Could you check a few things on this model? Use its own coordinates, in mm. A direction names the side the tool comes from. Coordinates: 2 decimals unless noted, no trailing zeros. Write each loop counter-clockwise with the first axis right and the second up, starting at its lowest first coordinate (ties: lowest second). Pieces come first, ordered by that corner, then holes. Notation, with made-up numbers: (82.25, -23) - (136.25, -23) arc R21 cw to (136.25, 15) - close; hole circle Ø8 at (50, 17). An arc over 180 degrees is marked (long way). Answer as a JSON object with one key per item and string values. Group by question number.
1) If we section it at B-B (y = 3): Write out the boundary of the cut face in (x, z).
2) Please list where these lines run through material, in increasing order: line 1 along Y through (x, z) = (-12.7, 138); line 2 along X through (y, z) = (-51, 87.5); line 3 along X through (y, z) = (-5, 118).
3) We'd pull the mould along Y, two halves only. Please class faces 1 (the flat face through (-24.3, -5.7, 38.1)), 2 (the flat face through (17.128, -105.736, 126.644)), 3 (the cylindrical face through (-0.586, -3.815, 18.783)): released by +Y, released by -Y, zero draft, split by the parting line, or undercut.
4) Will these pins go through, and if not, where does the flat tip stop? pin 1 Ø2 at (x, z) = (3.5, 68.5) entering from -Y; pin 2 Ø10 at (y, z) = (-62.5, 133.5) entering from -X; pin 3 Ø23 at (x, y) = (-12.7, 0) entering from +Z; pin 4 Ø1 at (x, z) = (-3, 30) entering from -Y.
5) If we section it at A-A (x = -12.7): Write out the boundary of the cut face in (y, z), plus the area to 3 significant figures.
6) On a 3-axis mill with a long thin cutter (end or side, diameter ignored), from which of +Z, -Z, +X, -X, +Y, -Y can I reach the whole of each face in a straight line? I mean faces 4 (the flat face through (6.159, -98.842, 126.644)), 5 (the flat face through (17.128, -105.736, 25.044)), 6 (the flat face through (1, -35, 0)), 7 (the flat face through (17.8, -108.83, 25.04)), 8 (the flat face through (-24.3, -5.7, 114.3)). Say none if no direction works.
7) If we section it at D-D (x = 7): Write out the boundary of the cut face in (y, z), plus the area to 3 significant figures.
8) If we section it at C-C (z = 111): Write out the boundary of the cut face in (x, y), plus the area to 3 significant figures.
```python
from build123d import *

# Parameters (mm, degrees)
SKETCH1_R           = 12.7
BOSS_EXTRUDE1_DEPTH = 152.4
CUT_EXTRUDE1_REACH  = 196.861
SKETCH2_W           = 50.8
SKETCH2_H           = 91.59656884
FILLET1_R           = 2.54
FILLET3_R           = 1.143
SKETCH4_W           = 76.2
SKETCH4_H           = 60.96
CUT_EXTRUDE3_DEPTH  = 38.1
SKETCH5_W           = 50.8
SKETCH5_H           = 6.992097594
BOSS_EXTRUDE2_DEPTH = 2.54


with BuildPart() as part:
    # Sketch1 → Boss-Extrude1 (new body)
    # profile 1 of 4: a face of its own
    with BuildSketch(Plane.XY):
        with BuildLine():
            Line((0, -8.424226968), (0, 0))
            Line((0, 0), (2.54, 0))
            ThreePointArc((2.54, 0), (-27.291189122, 4.399409051), (0, -8.424226968))
        make_face()
        with Locations(Location((-12.7, 0, 0), (0, 0, 180))):
            Circle(SKETCH1_R, mode=Mode.SUBTRACT)
    # profile 2 of 4: a face of its own
    with BuildSketch(Plane.XY):
        with BuildLine():
            Line((2.54, 0), (0, 0))
            Line((0, 0), (0, -8.424226968))
            ThreePointArc((0, -8.424226968), (1.891189122, -4.399409051), (2.54, 0))
        make_face()
    # profile 3 of 4: a face of its own
    with BuildSketch(Plane.XY):
        with BuildLine():
            ThreePointArc((2.54, 0), (1.891189122, -4.399409051), (0, -8.424226968))
            Line((0, -8.424226968), (0, -88.9))
            Line((0, -88.9), (2.54, -88.9))
            Line((2.54, -88.9), (2.54, 0))
        make_face()
    # profile 4 of 4: a face of its own
    with BuildSketch(Plane.XY):
        Polygon((22.969147698, -102.726355783), (10.424773969, -117.541831082), (0, -88.9), (2.54, -88.9), (11.22731164, -112.768192568), (21.023394812, -101.093675255), align=None)
    extrude(amount=BOSS_EXTRUDE1_DEPTH)

    # Sketch2 → Cut-Extrude1 (cut, up to next)
    with BuildSketch(Plane(origin=(2.54, 0, 0), x_dir=(0, 0, -1), z_dir=(1, 0, 0)), mode=Mode.PRIVATE) as cut_extrude1_sk1:
        with Locations((-76.2, -90.24828442)):
            Rectangle(SKETCH2_W, SKETCH2_H)
    cut_extrude1_tool1 = extrude(cut_extrude1_sk1.sketch, amount=CUT_EXTRUDE1_REACH, mode=Mode.PRIVATE) & part.part
    add(cut_extrude1_tool1.solids().sort_by_distance((2.54, -90.248284, 76.2))[0], mode=Mode.SUBTRACT)

    # Fillet1
    fillet1_edges = [part.edges().sort_by_distance(p)[0] for p in [
        (2.54, -88.9, 127),
        (11.22731164, -112.768192568, 127),
        (10.424773969, -117.541831082, 127),
        (2.54, -88.9, 25.4),
        (11.22731164, -112.768192568, 25.4),
        (10.424773969, -117.541831082, 25.4),
    ]]
    fillet(fillet1_edges, radius=FILLET1_R)

    # Fillet3
    fillet3_edges = [part.edges().sort_by_distance(p)[0] for p in [
        (21.023394812, -101.093675255, 127),
        (22.969147698, -102.726355783, 127),
        (21.023394812, -101.093675255, 25.4),
        (22.969147698, -102.726355783, 25.4),
    ]]
    fillet(fillet3_edges, radius=FILLET3_R)

    # Sketch4 → Cut-Extrude3 (cut)
    with BuildSketch(Plane.ZY):
        with Locations((76.2, 15.24)):
            Rectangle(SKETCH4_W, SKETCH4_H)
    extrude(amount=CUT_EXTRUDE3_DEPTH, mode=Mode.SUBTRACT)

    # Sketch5 → Boss-Extrude2 (add)
    with BuildSketch(Plane(origin=(2.54, 0, 0), x_dir=(0, 0, -1), z_dir=(1, 0, 0))):
        with Locations((-76.2, -92.382543848)):
            Rectangle(SKETCH5_W, SKETCH5_H)
    extrude(amount=BOSS_EXTRUDE2_DEPTH)


solid = part.part
```
Here are the results:
{
 "1": {"outline": "(-27.64, 0) - (-25.04, 0) - (-25.04, 38.1) - (-27.64, 38.1) - close; (-27.64, 114.3) - (-25.04, 114.3) - (-25.04, 152.4) - (-27.64, 152.4) - close; (-0.36, 0) - (2.24, 0) - (2.24, 152.4) - (-0.36, 152.4) - (-0.36, 114.3) - (0, 114.3) - (0, 38.1) - (-0.36, 38.1) - close"},
 "2": {"line 1": "y = -15.24 to -12.7, 12.7 to 15.24", "line 2": "x = 0 to 2.54", "line 3": "x = -27.1 to -24.37, -1.03 to 2.54"},
 "3": {"face 1": "zero draft", "face 2": "released by +Y", "face 3": "undercut"},
 "4": {"pin 1": "stops at y = -95.88", "pin 2": "stops at x = 0", "pin 3": "passes through", "pin 4": "stops at y = -12.15"},
 "5": {"outline": "(-15.24, 0) - (-12.7, 0) - (-12.7, 38.1) - (-15.24, 38.1) - close; (-15.24, 114.3) - (-12.7, 114.3) - (-12.7, 152.4) - (-15.24, 152.4) - close; (12.7, 0) - (15.24, 0) - (15.24, 38.1) - (12.7, 38.1) - close; (12.7, 114.3) - (15.24, 114.3) - (15.24, 152.4) - (12.7, 152.4) - close", "area": "387 mm²"},
 "6": {"face 4": "+Z, +Y", "face 5": "+Z, -Z, +Y", "face 6": "-Z, +X, -X, +Y, -Y", "face 7": "+Z, -Z, +X, -Y", "face 8": "-X, +Y, -Y"},
 "7": {"outline": "(-108.13, 0) - (-101.15, 0) - (-101.15, 50.8) - (-108.13, 50.8) - close; (-108.13, 101.6) - (-101.15, 101.6) - (-101.15, 152.4) - (-108.13, 152.4) - close", "area": "709 mm²"},
 "8": {"outline": "(0, -88.9) - (8.93, -113.43) arc R2.54 ccw to (13.25, -114.2) - (22.23, -103.6) arc R1.14 ccw to (22.09, -101.99) - (21.9, -101.83) arc R1.14 ccw to (20.29, -101.97) - (14.06, -109.4) arc R2.54 cw to (9.72, -108.63) - (2.69, -89.32) arc R2.54 cw to (2.54, -88.45) - (2.54, 0) arc R15.24 ccw to (0, 8.42) - close", "area": "350 mm²"}
}
